Design review of the part built by this model. Coordinates are the model's own, in mm. Face numbers are marked on the shaded views. A direction names the side the tool comes from. Round coordinates to 2 decimals unless told otherwise and drop trailing zeros. Write each loop counter-clockwise with the first axis right and the second up, starting at its lowest first coordinate (ties: lowest second). Pieces come first, ordered by that corner, then holes. Notation, with made-up numbers: (70, 67.5) -> (82, 67.5) arc R27 ccw to (82, 106.5) -> close; hole circle Ø4 at (35.25, -3.5). An arc over 180 degrees is marked (long way). Write item = value, one per line. Start each with the question number.
Item 1: Add section B-B, the plane z = 21.75. State the section outline as (x, y) points.
Item 2: Machinability: for the marked faces 1, 2 and 3, which of the approach directions +Z, -Z, +X, -X, +Y, -Y give a long, thin tool a straight path to every point of the face, cutting with its end or side? Answer none if there is none.
Item 3: Mouldability with a two-part tool opening along Y and no side actions: class the marked faces 4, 5 and 6 as released by +Y, released by -Y, zero draft, split by the parting line, or undercut.
Item 4: For pin 1 Ø10 at (x, z) = (-20, 16.5) entering from -Y; pin 2 Ø24 at (x, y) = (0, 0) entering from -Z; pin 3 Ø2 at (x, z) = (-10.5, 13) entering from +Y; pin 4 Ø8 at (y, z) = (-16, 13) entering from -X, all flat-tipped, find the tip position at first contact; note any pin that passes through.
Item 5: To check wall thickness, follow L1, parallel to X at y = 0, z = 12.05; L2, parallel to Y at x = 0, z = 18; L3, parallel to X at y = 0, z = 13.75. State the ranges of each line that lie inside material, in increasing order.
Item 6: Add section D-D, the plane z = 28. State the section outline as (x, y) points.
from build123d import *

# Parameters (mm, degrees)
F3_DEPTH = 25


with BuildPart() as f1:
    # F0 (on Front) → F1 (revolve)
    with BuildSketch(Plane.XZ):
        Polygon((15, 5), (15, 0), (22.5, 0), (22.5, 17), (21, 17), (21, 20), (30, 20), (30, 30), (15, 30), (15, 29), (18, 25), (15, 25), (15, 16), (18, 16), (18, 13), (15, 13), (15, 8), (17, 8), (17, 5), align=None)
    revolve(axis=Axis((0, 0, 16.846085), (0, 0, -1)))

    # F2 (on face) → F3 (intersect)
    with BuildSketch(Plane.XY.offset(30)):
        Polygon((0, -31.176915), (27, -15.588457), (27, 15.588457), (0, 31.176915), (-27, 15.588457), (-27, -15.588457), align=None)
    extrude(amount=-F3_DEPTH, mode=Mode.INTERSECT)


solid = f1.part
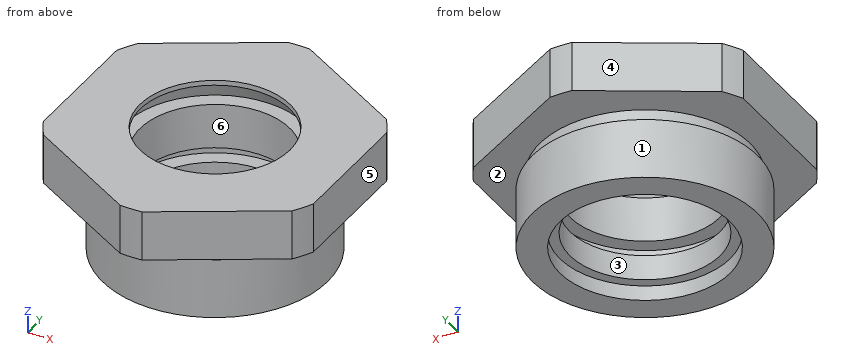
Result set:
q1.outline = (-27, -13.08) arc R30 ccw to (-24.82, -16.84) -> (-2.18, -29.92) arc R30 ccw to (2.18, -29.92) -> (24.82, -16.84) arc R30 ccw to (27, -13.08) -> (27, 13.08) arc R30 ccw to (24.82, 16.84) -> (2.18, 29.92) arc R30 ccw to (-2.18, 29.92) -> (-24.82, 16.84) arc R30 ccw to (-27, 13.08) -> close; hole circle Ø30 at (0, 0)
q2.face_1 = -Z
q2.face_2 = none
q2.face_3 = +Z, -Z
q3.face_4 = released by +Y
q3.face_5 = zero draft
q3.face_6 = undercut
q4.pin_1 = -21.69
q4.pin_2 = through
q4.pin_3 = 20.4
q4.pin_4 = -19.03
q5.L1 = -22.5 to -15, 15 to 22.5
q5.L2 = -21 to -15, 15 to 21
q5.L3 = -22.5 to -18, 18 to 22.5
q6.outline = (-27, -13.08) arc R30 ccw to (-24.82, -16.84) -> (-2.18, -29.92) arc R30 ccw to (2.18, -29.92) -> (24.82, -16.84) arc R30 ccw to (27, -13.08) -> (27, 13.08) arc R30 ccw to (24.82, 16.84) -> (2.18, 29.92) arc R30 ccw to (-2.18, 29.92) -> (-24.82, 16.84) arc R30 ccw to (-27, 13.08) -> close; hole circle Ø31.5 at (0, 0)
